Design review of the part built by this model. Coordinates are the model's own, in mm. Face numbers are marked on the shaded views. A direction names the side the tool comes from. Coordinates: 2 decimals unless noted, no trailing zeros. Write each loop counter-clockwise with the first axis right and the second up, starting at its lowest first coordinate (ties: lowest second). Pieces come first, ordered by that corner, then holes.
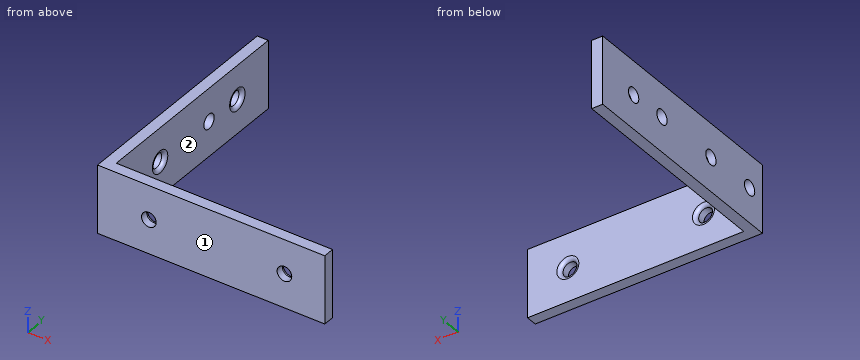
```python
from build123d import *

# Parameters (mm, degrees)
SKETCH1_W           = 62
SKETCH1_H           = 62
BOSS_EXTRUDE1_DEPTH = 18.5
SKETCH2_W           = 59
SKETCH2_H           = 59
CUT_EXTRUDE1_DEPTH  = 18.5
SKETCH3_R           = 2
CUT_EXTRUDE2_DEPTH  = 3
SKETCH4_R           = 2
CUT_EXTRUDE3_DEPTH  = 3
FILLET1_R           = 1
FILLET2_R           = 1
SKETCH5_R           = 2
CUT_EXTRUDE4_DEPTH  = 3
SKETCH6_R           = 2
CUT_EXTRUDE5_DEPTH  = 3
FILLET3_R           = 1
FILLET4_R           = 1
SKETCH7_R           = 2
CUT_EXTRUDE6_DEPTH  = 3
SKETCH8_R           = 2
CUT_EXTRUDE7_DEPTH  = 3


with BuildPart() as part:
    # Sketch1 → Boss-Extrude1 (new body)
    with BuildSketch(Plane.XY):
        Rectangle(SKETCH1_W, SKETCH1_H)
    extrude(amount=BOSS_EXTRUDE1_DEPTH)

    # Sketch2 → Cut-Extrude1 (cut)
    with BuildSketch(Plane.XY.offset(18.5)):
        with Locations((1.5, 1.5)):
            Rectangle(SKETCH2_W, SKETCH2_H)
    extrude(amount=-CUT_EXTRUDE1_DEPTH, mode=Mode.SUBTRACT)

    # Sketch3 → Cut-Extrude2 (cut)
    with BuildSketch(Plane(origin=(0, -28, 0), x_dir=(1, 0, 0), z_dir=(0, 1, 0))):
        with Locations((-17, -9.25)):
            Circle(SKETCH3_R)
    extrude(amount=-CUT_EXTRUDE2_DEPTH, mode=Mode.SUBTRACT)

    # Sketch4 → Cut-Extrude3 (cut)
    with BuildSketch(Plane(origin=(0, -28, 0), x_dir=(1, 0, 0), z_dir=(0, 1, 0))):
        with Locations((20, -9.25)):
            Circle(SKETCH4_R)
    extrude(amount=-CUT_EXTRUDE3_DEPTH, mode=Mode.SUBTRACT)

    # Fillet1
    fillet1_edges = [part.edges().sort_by_distance(p)[0] for p in [
        (18, -28, 9.25),
    ]]
    fillet(fillet1_edges, radius=FILLET1_R)

    # Fillet2
    fillet2_edges = [part.edges().sort_by_distance(p)[0] for p in [
        (-19, -28, 9.25),
    ]]
    fillet(fillet2_edges, radius=FILLET2_R)

    # Sketch5 → Cut-Extrude4 (cut)
    with BuildSketch(Plane(origin=(-28, 0, 0), x_dir=(0, 0, -1), z_dir=(1, 0, 0))):
        with Locations((-9.25, -11)):
            Circle(SKETCH5_R)
    extrude(amount=-CUT_EXTRUDE4_DEPTH, mode=Mode.SUBTRACT)

    # Sketch6 → Cut-Extrude5 (cut)
    with BuildSketch(Plane(origin=(-28, 0, 0), x_dir=(0, 0, -1), z_dir=(1, 0, 0))):
        with Locations((-9.25, 19)):
            Circle(SKETCH6_R)
    extrude(amount=-CUT_EXTRUDE5_DEPTH, mode=Mode.SUBTRACT)

    # Fillet3
    fillet3_edges = [part.edges().sort_by_distance(p)[0] for p in [
        (-28, 19, 11.25),
    ]]
    fillet(fillet3_edges, radius=FILLET3_R)

    # Fillet4
    fillet4_edges = [part.edges().sort_by_distance(p)[0] for p in [
        (-28, -11, 11.25),
    ]]
    fillet(fillet4_edges, radius=FILLET4_R)

    # Sketch7 → Cut-Extrude6 (cut)
    with BuildSketch(Plane(origin=(-28, 0, 0), x_dir=(0, 0, -1), z_dir=(1, 0, 0))):
        with Locations((-9.5, -26)):
            Circle(SKETCH7_R)
    extrude(amount=-CUT_EXTRUDE6_DEPTH, mode=Mode.SUBTRACT)

    # Sketch8 → Cut-Extrude7 (cut)
    with BuildSketch(Plane(origin=(-28, 0, 0), x_dir=(0, 0, -1), z_dir=(1, 0, 0))):
        with Locations((-9.5, 8)):
            Circle(SKETCH8_R)
    extrude(amount=-CUT_EXTRUDE7_DEPTH, mode=Mode.SUBTRACT)


solid = part.part
```
(1) Wall thickness on line 1 (Y direction, x = -29.5, z = 9.25); line 2 (Z direction, x = -29.9, y = -26); line 3 (X direction, y = -30.25, z = 9.25): over which ranges is each line inside the solid? List them lowest first.
(2) Consider section B-B (x = 20). Give the boundary of the cut face in (y, z), plus the area to 3 significant figures.
(3) Consider section A-A (y = 8). Give the boundary of the cut face in (x, z).
(4) For the marked faces 1 and 2, list the 3-axis set-ups (+Z, -Z, +X, -X, +Y, -Y) from which the entire face can be reached by the end or side of a thin tool; tool diameter is ignored.
(5) Insertion check: pin 1 Ø2 at (x, z) = (-3.5, 15) entering from +Y; pin 2 Ø3 at (x, z) = (-17, 9.25) entering from -Y. Each pin has a flat end and moves straight along its axis. Give the tip position at first contact, or say it passes through.
(6) Consider section C-C (z = 17.75). Give the boundary of the cut face in (x, y), plus the area to 3 significant figures.
Results:
1. line 1: y = -31 to -27.98, -24.02 to -13, -9 to 6.02, 9.98 to 17, 21 to 31
1. line 2: z = 0 to 7.5, 11.5 to 18.5
1. line 3: x = -31 to -19, -15 to 18, 22 to 31
2. outline: (-31, 0) - (-28, 0) - (-28, 6.25) arc R1 ccw to (-29, 7.25) - (-31, 7.25) - close; (-31, 11.25) - (-29, 11.25) arc R1 ccw to (-28, 12.25) - (-28, 18.5) - (-31, 18.5) - close
2. area: 43.1 mm2
3. outline: (-31, 0) - (-28, 0) - (-28, 7.5) - (-31, 7.5) - close; (-31, 11.5) - (-28, 11.5) - (-28, 18.5) - (-31, 18.5) - close
4. face 1: +Z, -Z, +X, -X, -Y
4. face 2: +Z, -Z, +X, +Y
5. pin 1: stops at y = -28
5. pin 2: passes through
6. outline: (-31, -31) - (31, -31) - (31, -28) - (-28, -28) - (-28, 31) - (-31, 31) - close
6. area: 363 mm2
